Source: CAD feature listing. Evaluate the final solid. Frame: model axes, mm. A direction names the side the tool comes from. Give positions to 0.01 mm unless a question says otherwise; leave off trailing zeros. Order: outer loops, then holes, each group sorted by start corner. A loop starts at its lowest first (then second) coordinate and runs counter-clockwise, first axis right, second up. Notation, with made-up numbers: M -0.75,69 L 51.25,69 A26 cw 51.25,100 Z; hole C 33,82 d11. An arc over 180 degrees is marked long. Answer in a Markdown table with one row per item. Add a question column.
(1) Mould query, pull axis Z, two halves, no side actions, for faces 1 (the face through (0.8, -3.6, 4.6)), 2 (the face through (2, 0, 0)), 3 (the face through (1.5, -3.85, 1.5)). Classes: pulls with the +Z half, pulls with the -Z half, needs draft (parallel to the pull), parting line crosses it, or undercut.
(2) Section query C-C, the plane x = 4.25. Return loops of the section in (y, z).
(3) Section query B-B, the plane y = -2.5. Return loops of the section in (x, z), plus the area to 3 significant figures.
(4) Set-up query: faces 4 (the face through (1.6, 3.85, 1.5)), 5 (the face through (1.7, 0, 3)). Return all of +Z, -Z, +X, -X, +Y, -Y with unobstructed straight access to the full face (end or side cutting, diameter ignored); none if empty.
(5) Material intervals for line 1 along X through (y, z) = (-2, 1.95); line 2 along Y through (x, z) = (1.05, 4.65), sorted ascending.
(6) Section query A-A, the plane z = 4.4. Return loops of the section in (x, y), plus the area to 4 significant figures.
(7) Pin query (flat end, axial travel): P1, Ø0.9, axis at y = 0.5, z = 3, coming from the +X side; P2, Ø2.5, axis at x = 4, y = 1.5, coming from the +Z side; P3, Ø1.5, axis at x = 2.5, z = 4, coming from the -Y side. Return the tip coordinate at first contact, or that it passes through.
from build123d import *

# Parameters (mm, degrees)
FLUSH_ROOF_LENS_T1_7_CLEARANCE0_15_DEPTH = 1.7
FLUSH_SIDE_LENS_T1_7_CLEARANCE0_15_DEPTH = 1.7


with BuildPart() as part:
    # 草图1 → Flush_roof_lens_T1.7_clearance0.15 (new body)
    with BuildSketch(Plane.XY):
        with BuildLine():
            Line((0, -3.85), (4, -3.85))
            ThreePointArc((4, -3.85), (4.601040764, -3.601040764), (4.85, -3))
            Line((4.85, -3), (4.85, 3))
            ThreePointArc((4.85, 3), (4.601040764, 3.601040764), (4, 3.85))
            Line((4, 3.85), (0, 3.85))
            Line((0, 3.85), (0, -3.85))
        make_face()
    extrude(amount=FLUSH_ROOF_LENS_T1_7_CLEARANCE0_15_DEPTH)

    # 草图2 → Flush_side_lens_T1.7_clearance0.15 (add)
    with BuildSketch(Plane(origin=(0, 0, 0), x_dir=(0, 0, -1), z_dir=(1, 0, 0))):
        with BuildLine():
            Line((0, -3.85), (0, 3.85))
            Line((0, 3.85), (-4, 3.85))
            ThreePointArc((-4, 3.85), (-4.601040764, 3.601040764), (-4.85, 3))
            Line((-4.85, 3), (-4.85, -3))
            ThreePointArc((-4.85, -3), (-4.601040764, -3.601040764), (-4, -3.85))
            Line((-4, -3.85), (0, -3.85))
        make_face()
    extrude(amount=FLUSH_SIDE_LENS_T1_7_CLEARANCE0_15_DEPTH)


solid = part.part
Values follow:
| question | item | result |
|---|---|---|
| 1 | face 1 | pulls with the +Z half |
| 1 | face 2 | pulls with the -Z half |
| 1 | face 3 | needs draft |
| 2 | outline | M -3.81,0 L 3.81,0 L 3.81,1.7 L -3.81,1.7 Z |
| 3 | outline | M 0,0 L 4.85,0 L 4.85,1.7 L 1.7,1.7 L 1.7,4.85 L 0,4.85 Z |
| 3 | area | 13.6 mm² |
| 4 | face 4 | +Z, -Z, +X, -X, +Y |
| 4 | face 5 | +Z, +X, +Y, -Y |
| 5 | line 1 | x = 0 to 1.7 |
| 5 | line 2 | y = -3.55 to 3.55 |
| 6 | outline | M 0,-3.75 L 1.7,-3.75 L 1.7,3.75 L 0,3.75 Z |
| 6 | area | 12.75 mm² |
| 7 | P1 | stops at x = 1.7 |
| 7 | P2 | stops at z = 1.7 |
| 7 | P3 | passes through |
